```python
from build123d import *

# Parameters (mm, degrees)
SKETCH1_W           = 25.4
SKETCH1_H           = 38.1
SKETCH1_W_2         = 19.05
SKETCH1_H_2         = 31.75
BOSS_EXTRUDE1_DEPTH = 1320.8
SKETCH2_R           = 3.175
CUT_EXTRUDE1_DEPTH  = 3.175


with BuildPart() as part:
    # Sketch1 → Boss-Extrude1 (new body)
    with BuildSketch(Plane(origin=(0, 0, 0), x_dir=(1, 0, 0), z_dir=(0, 1, 0))):
        Rectangle(SKETCH1_W, SKETCH1_H)
        Rectangle(SKETCH1_W_2, SKETCH1_H_2, mode=Mode.SUBTRACT)
    extrude(amount=BOSS_EXTRUDE1_DEPTH)

    # Sketch2 → Cut-Extrude1 (cut)
    with BuildSketch(Plane.ZY.offset(12.7)):
        with Locations((0, 25.4)):
            Circle(SKETCH2_R)
        with Locations((0, 228.6)):
            Circle(SKETCH2_R)
    cut_extrude1 = extrude(amount=-CUT_EXTRUDE1_DEPTH, mode=Mode.SUBTRACT)

    # Mirror1: Cut-Extrude1 across plane
    add(cut_extrude1.mirror(Plane(origin=(0, 0, 0), x_dir=(0, 0, 1), z_dir=(1, 0, 0))), mode=Mode.SUBTRACT)


solid = part.part
```
Work out the finished part from the listing and answer in its coordinate system (mm). A direction names the side the tool comes from. Round coordinates to 2 decimals unless told otherwise and drop trailing zeros. Write each loop counter-clockwise with the first axis right and the second up, starting at its lowest first coordinate (ties: lowest second). Pieces come first, ordered by that corner, then holes.
1) Flat-ended cylindrical pins translate along their axes: P1, Ø5.5, axis at y = 228.6, z = 0, coming from the -X side; P2, Ø7.5, axis at y = 25.4, z = 0, coming from the +X side. Find the tip coordinate at first contact, or state that the pin passes through.
2) Determine the mould class of faces 1 (the face through (0, 651, -19.05)), 2 (the face through (-9.525, 651, 0)), 3 (the face through (12.7, 651, 0)) for opening direction X: pulls with the +X half, pulls with the -X half, needs draft (parallel to the pull), parting line crosses it, or undercut.
3) A cutting plane is placed at A-A on y = 445. Determine the outline of the cut face in (x, z) (3 decimals).
4) Which of the six approach directions +Z, -Z, +X, -X, +Y, -Y give full straight-line access (tool end or side, diameter ignored) to faces 4 (the face through (9.525, 651, 0)), 5 (the face through (0, 651, 19.05))?
5) Consider probe 1 along Y at (x, z) = (11.35, 0) (3 decimals); probe 2 along Z at (x, y) = (4.75, 768.5) (3 decimals); probe 3 along Z at (x, y) = (-11.5, 228.6) (3 decimals). Determine where each line is inside the solid, lowest interval first.
6) A cutting plane is placed at B-B on x = -2. Determine the outline of the cut face in (y, z) (3 decimals), and give its area (3 significant figures).
Entries:
1. P1: passes through
1. P2: stops at x = 12.7
2. face 1: needs draft
2. face 2: undercut
2. face 3: pulls with the +X half
3. outline: (-12.7, -19.05) - (12.7, -19.05) - (12.7, 19.05) - (-12.7, 19.05) - close; hole (-9.525, -15.875) - (9.525, -15.875) - (9.525, 15.875) - (-9.525, 15.875) - close
4. face 4: +Y, -Y
4. face 5: +Z, +X, -X, +Y, -Y
5. probe 1: y = 0 to 22.225, 28.575 to 225.425, 231.775 to 1320.8
5. probe 2: z = -19.05 to -15.875, 15.875 to 19.05
5. probe 3: z = -19.05 to -3.175, 3.175 to 19.05
6. outline: (0, -19.05) - (1320.8, -19.05) - (1320.8, -15.875) - (0, -15.875) - close; (0, 15.875) - (1320.8, 15.875) - (1320.8, 19.05) - (0, 19.05) - close
6. area: 8,390 mm2
